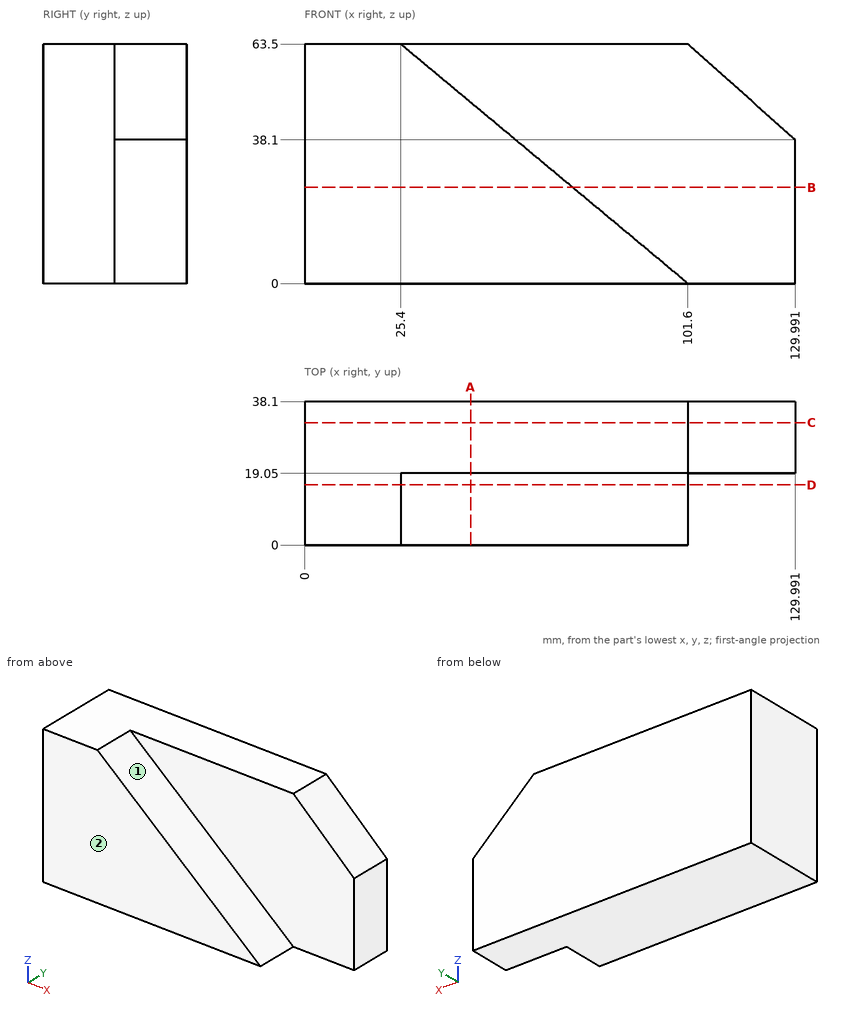
Source: three-view drawing plus pictorial views. Frame: mm from the lowest corner of the part. A direction names the side the tool comes from. Coordinates: 2 decimals unless noted, no trailing zeros. Write each loop counter-clockwise with the first axis right and the second up, starting at its lowest first coordinate (ties: lowest second). Pieces come first, ordered by that corner, then holes. Notation, with made-up numbers: (43, 85) - (101, 85) arc R27 ccw to (101, 109) - close; hole circle Ø3 at (20, -7.75). An arc over 180 degrees is marked (long way). Answer as a JSON object with one key per item and string values.
Q1. Set-up query: the marked faces 1 and 2. Return all of +Z, -Z, +X, -X, +Y, -Y with unobstructed straight access to the full face (end or side cutting, diameter ignored); none if empty.
Ans:
{"face 1": "+Z, +X, -Y", "face 2": "+Z, -Z, +X, -X, -Y"}
Q2. Section query A-A, the plane x = 44. Output: boundary loops of the cut face in (y, z), plus the area to 3 significant figures.
Ans:
{"outline": "(0, 0) - (38.1, 0) - (38.1, 63.5) - (19.05, 63.5) - (19.05, 48) - (0, 48) - close", "area": "2,120 mm2"}
Q3. Section query C-C, the plane y = 32.5. Output: boundary loops of the cut face in (x, z).
Ans:
{"outline": "(0, 0) - (129.99, 0) - (129.99, 38.1) - (101.6, 63.5) - (0, 63.5) - close"}
Q4. Section query B-B, the plane z = 25.5. Output: boundary loops of the cut face in (x, y).
Ans:
{"outline": "(0, 0) - (71, 0) - (71, 19.05) - (129.99, 19.05) - (129.99, 38.1) - (0, 38.1) - close"}
Q5. Material intervals for line 1 (Y direction, x = 122.5, z = 6.5); line 2 (X direction, y = 31.5, z = 49.5); line 3 (X direction, y = 17, z = 26), sorted ascending. Write a range as [from, to].
Ans:
{"line 1": "y = [19.05, 38.1]", "line 2": "x = [0, 117.25]", "line 3": "x = [0, 70.4]"}
Q6. First-contact query: pin 1 Ø1.5 at (x, z) = (86.5, 13.5) entering from -Y. Flat tip, straight axial feed; report the tip coordinate or a pass-through.
Ans:
{"pin 1": "stops at y = 0"}
Q7. Section query D-D, the plane y = 16. Output: boundary loops of the cut face in (x, z).
Ans:
{"outline": "(0, 0) - (101.6, 0) - (25.4, 63.5) - (0, 63.5) - close"}
